from build123d import *

# Parameters (mm, degrees)
SKETCH_1_R              = 6
SKETCH_1_R_2            = 2.6
EXTRUDE_1_DEPTH         = 22
CUT_EXTRUDE_START       = -12
CUT_EXTRUDE_1_OUTLINE_R = 6
CUT_EXTRUDE_1_DEPTH     = 12
FILLET_1_R              = 5


# Read off the part's stored shape, not the designer's step: 切除-拉伸1
with BuildPart() as part:
    # 草图1 → 凸台-拉伸1 (new body)
    with BuildSketch(Plane.XY):
        with BuildLine():
            Line((24.04705584, 21.941390991), (25.62631028, -1.269568576))
            add(Edge.make_bspline(
                [(25.62631028, -1.269568576), (30.294741582, 4.490329629), (34.848985416, 10.341994574), (43.840833171, 22.214968329), (48.277316557, 28.236694952), (52.668077763, 34.291262241)],
                knots=[0.751086715, 0.751086715, 0.751086715, 0.751086715, 0.875, 0.875, 1, 1, 1, 1], degree=3))
            add(Edge.make_bspline(
                [(52.668077763, 34.291262241), (54.385569076, 36.659627804), (56.095877797, 39.033185186), (58.65356822, 42.599078019), (59.503877121, 43.78931812), (61.206685795, 46.168192958), (62.060572053, 47.355980663), (62.923151952, 48.537325445)],
                knots=[0, 0, 0, 0, 12.867122322, 12.867122322, 19.300683483, 19.300683483, 25.734244644, 25.734244644, 25.734244644, 25.734244644], degree=3))
            add(Edge.make_bspline(
                [(62.923151952, 48.537325445), (63.691030086, 49.593267388), (64.385737457, 50.528608987), (65.152866174, 51.561457391), (65.870104463, 52.500349083), (66.644032214, 53.513449395), (67.382538536, 54.446906012), (68.169071386, 55.441067159), (68.929366855, 56.362602713)],
                knots=[0, 0, 0, 0.25, 0.25, 0.5, 0.5, 0.75, 0.75, 1, 1, 1], degree=2))
            add(Edge.make_bspline(
                [(68.929366855, 56.362602713), (68.939807825, 56.376913703), (68.94904286, 56.392240586)],
                knots=[0.088106579, 0.088106579, 0.088106579, 0.143786066, 0.143786066, 0.143786066], degree=2, weights=[1, 0.999612499, 1]))
            Line((68.94904286, 56.392240586), (73.182530774, 63.58271012))
            Line((73.182530774, 63.58271012), (77.6764923, 67.17962487))
            ThreePointArc((77.6764923, 67.17962487), (78.379967095, 67.75128437), (79.091839453, 68.312452009))
            Line((79.091839453, 68.312452009), (103.36876376, 87.743421018))
            add(Edge.make_bspline(
                [(103.36876376, 87.743421018), (103.794913212, 88.083498112), (104.14591982, 88.500209303), (104.495810247, 88.915595377), (104.757584433, 89.390611784), (105.019785316, 89.866402479), (105.18387744, 90.383514181), (105.347603834, 90.89947334), (105.407790685, 91.436682712), (105.468371762, 91.977410832), (105.422168005, 92.518813243), (105.376170251, 93.057801763), (105.226513558, 93.576866403), (105.075866476, 94.099366077), (104.826403144, 94.581721125), (104.577389608, 95.06320646), (104.239613139, 95.486702432)],
                knots=[0, 0, 0, 0.125, 0.125, 0.25, 0.25, 0.375, 0.375, 0.5, 0.5, 0.625, 0.625, 0.75, 0.75, 0.875, 0.875, 1, 1, 1], degree=2))
            Line((104.239613139, 95.486702432), (102.10787197, 98.150082549))
            add(Edge.make_bspline(
                [(102.10787197, 98.150082549), (101.662660323, 98.707408746), (101.134816221, 99.186660834), (100.605787322, 99.666988651), (100.007698858, 100.056631193), (99.413800036, 100.443544268), (98.766951597, 100.73157288), (98.115443256, 101.021676452), (97.426848492, 101.204456829), (96.741213417, 101.386451586), (96.036172435, 101.457788474), (95.327397899, 101.529503128), (94.616958411, 101.487928839), (93.907956416, 101.446438671), (93.215156177, 101.29350915), (92.520746602, 101.140224382), (91.859708878, 100.879055504)],
                knots=[0, 0, 0, 0.125, 0.125, 0.25, 0.25, 0.375, 0.375, 0.5, 0.5, 0.625, 0.625, 0.75, 0.75, 0.875, 0.875, 1, 1, 1], degree=2))
            Line((91.859708878, 100.879055504), (81.022663549, 97.937140274))
            Line((81.022663549, 97.937140274), (66.880013026, 92.33227511))
            add(Edge.make_bspline(
                [(66.880013026, 92.33227511), (65.373977149, 91.735592871), (64.00578846, 90.868278931), (62.646323986, 90.006495393), (61.470305816, 88.907497765), (60.292351586, 87.806690876), (59.339427675, 86.506195587), (58.383073515, 85.201018894), (57.686838347, 83.740417625)],
                knots=[0, 0, 0, 0.25, 0.25, 0.5, 0.5, 0.75, 0.75, 1, 1, 1], degree=2))
            add(Edge.make_bspline(
                [(57.686838347, 83.740417625), (56.095548431, 80.401632953), (54.518583687, 77.162280014)],
                knots=[0, 0, 0, 1, 1, 1], degree=2))
            add(Edge.make_bspline(
                [(54.518583687, 77.162280014), (53.763269837, 75.610969128), (52.999745837, 74.063699923), (51.467519232, 70.971710828), (50.697291265, 69.427763476), (49.146563784, 66.345016376), (48.366275895, 64.806128726), (46.794629467, 61.734063391), (46.003946156, 60.200522916), (45.205011248, 58.67121375)],
                knots=[0, 0, 0, 0, 0.25, 0.25, 0.5, 0.5, 0.75, 0.75, 1, 1, 1, 1], degree=3))
            add(Edge.make_bspline(
                [(45.205011248, 58.67121375), (41.847412181, 52.245521434), (38.381271035, 45.876195204), (31.340232317, 33.621328767), (27.77883413, 27.726649653), (24.04705584, 21.941390991)],
                knots=[0, 0, 0, 0, 0.125, 0.125, 0.243696274, 0.243696274, 0.243696274, 0.243696274], degree=3))
        make_face()
        with Locations((94.625559773, 92.089088396)):
            Circle(SKETCH_1_R, mode=Mode.SUBTRACT)
        with Locations((68.602677697, 77.162280014)):
            Circle(SKETCH_1_R, mode=Mode.SUBTRACT)
        with Locations((33.14705584, 20.777472123)):
            Circle(SKETCH_1_R_2, mode=Mode.SUBTRACT)
        with Locations((57.169835175, 58.366266824)):
            Circle(SKETCH_1_R_2, mode=Mode.SUBTRACT)
    extrude(amount=EXTRUDE_1_DEPTH)

    # 切除-拉伸1 outline → 切除-拉伸1 (cut)
    with BuildSketch(Plane.XY.offset(22).offset(CUT_EXTRUDE_START)):
        with BuildLine():
            add(Edge.make_bspline(
                [(57.686838346, 83.740417623), (56.09554843, 80.401632953), (54.518583688, 77.162280014)],
                knots=[0.494428836, 0.494428836, 0.494428836, 0.494587311, 0.494587311, 0.494587311], degree=2))
            Line((54.518583688, 77.162280014), (73.182530774, 63.58271012))
            Line((73.182530774, 63.58271012), (77.6764923, 67.17962487))
            ThreePointArc((77.6764923, 67.17962487), (78.379967095, 67.75128437), (79.091839453, 68.312452009))
            Line((79.091839453, 68.312452009), (103.36876376, 87.743421018))
            add(Edge.make_bspline(
                [(103.36876376, 87.743421018), (103.794913212, 88.083498112), (104.14591982, 88.500209303), (104.495810247, 88.915595377), (104.757584433, 89.390611784), (105.019785316, 89.866402479), (105.18387744, 90.383514181), (105.347603834, 90.89947334), (105.407790685, 91.436682712), (105.468371762, 91.977410832), (105.422168005, 92.518813243), (105.376170251, 93.057801763), (105.226513558, 93.576866403), (105.075866476, 94.099366077), (104.826403144, 94.581721125), (104.577389608, 95.06320646), (104.239613139, 95.486702432)],
                knots=[0, 0, 0, 0.125, 0.125, 0.25, 0.25, 0.375, 0.375, 0.5, 0.5, 0.625, 0.625, 0.75, 0.75, 0.875, 0.875, 1, 1, 1], degree=2))
            Line((104.239613139, 95.486702432), (102.10787197, 98.150082549))
            add(Edge.make_bspline(
                [(102.10787197, 98.150082549), (101.662660323, 98.707408746), (101.134816221, 99.186660834), (100.605787322, 99.666988651), (100.007698858, 100.056631193), (99.413800036, 100.443544268), (98.766951597, 100.73157288), (98.115443256, 101.021676452), (97.426848492, 101.204456829), (96.741213417, 101.386451586), (96.036172435, 101.457788474), (95.327397899, 101.529503128), (94.616958411, 101.487928839), (93.907956416, 101.446438671), (93.215156177, 101.29350915), (92.520746602, 101.140224382), (91.859708878, 100.879055504)],
                knots=[0, 0, 0, 0.125, 0.125, 0.25, 0.25, 0.375, 0.375, 0.5, 0.5, 0.625, 0.625, 0.75, 0.75, 0.875, 0.875, 1, 1, 1], degree=2))
            Line((91.859708878, 100.879055504), (81.022663549, 97.937140274))
            Line((81.022663549, 97.937140274), (66.880013026, 92.33227511))
            add(Edge.make_bspline(
                [(66.880013026, 92.33227511), (65.373977149, 91.735592871), (64.00578846, 90.868278931), (62.646323986, 90.006495393), (61.470305816, 88.907497765), (60.292351586, 87.806690876), (59.339427675, 86.506195587), (58.383073515, 85.201018894), (57.686838346, 83.740417623)],
                knots=[0, 0, 0, 0.25, 0.25, 0.5, 0.5, 0.75, 0.75, 1, 1, 1], degree=2))
        make_face()
        with Locations((68.602677697, 77.162280014)):
            Circle(CUT_EXTRUDE_1_OUTLINE_R, mode=Mode.SUBTRACT)
        with Locations((94.625559773, 92.089088396)):
            Circle(CUT_EXTRUDE_1_OUTLINE_R, mode=Mode.SUBTRACT)
    extrude(amount=CUT_EXTRUDE_1_DEPTH, mode=Mode.SUBTRACT)

    # 圆角1
    fillet_1_edges = [part.edges().sort_by_distance(p)[0] for p in [
        (73.182530774, 63.58271012, 16),
    ]]
    fillet(fillet_1_edges, radius=FILLET_1_R)
    # the kernel refuses this fillet: 5 mm, written as the material it takes off along each edge
    with BuildSketch(Plane(origin=(54.518583687, 77.162280014, 10), x_dir=(0.8086167393984858, -0.5883357619289866, 0), z_dir=(0, 0, 1))) as fillet_1_2_piece_1:
        with BuildLine():
            CenterArc((5.939761688, -5), FILLET_1_R, 89.999999998, 99.633547548)
            Line((1.010270575, -5.836730169), (0.911680753, -5.853464772))
            ThreePointArc((0.911680753, -5.853464772), (0.412045155, -2.934442011), (-0.098457006, -0.017499087))
            Line((-0.098457006, -0.017499087), (0, 0.1))
            Line((0, 0.1), (5.939761688, 0.1))
            Line((5.939761688, 0.1), (5.939761688, 0))
        make_face()
    extrude(amount=26.849404219, mode=Mode.SUBTRACT)


solid = part.part
Geometry: final body of the model. Coordinates: model frame, mm. A direction names the side the tool comes from. Round coordinates to 2 decimals unless told otherwise and drop trailing zeros. Loops run counter-clockwise (first coordinate to the right, second up) from the corner with the lowest first, then second, coordinate; pieces in that order, holes last. Notation, with made-up numbers: M 4.5,86 L 56.5,86 A10 cw 56.5,101 Z; hole C 81.25,1 d11. An arc over 180 degrees is marked long. Put each result on its own line as item: value. Start each with the question number.
(1) Set-up query: faces 5 (the face through (64.35, 70.01, 15.92)), 6 (the face through (55.11, 56.78, 10.85)), 7 (the face through (55.248, 74.495, 15.916)). Return all of +Z, -Z, +X, -X, +Y, -Y with unobstructed straight access to the full face (end or side cutting, diameter ignored); none if empty.
(2) Draft query along X for faces 1 (the face through (100.35, 93.89, 4.93)), 2 (the face through (86.52, 99.43, 4.93)), 3 (the face through (71.477, 63.176, 16.084)), 4 (the face through (79, 84, 10)). Return one class per face: +X half, -X half, draft (parallel to the pull), parting line (faces both ways), or undercut.
(3) Section query A-A (z = 18). State how many separate pieces and enclosed holes the cut face has, then the cut area to 3 significant figures.
(4) Contact query for flat-ended pins moving along their axis: pin 1 Ø2 at (x, z) = (58.5, 17) entering from -Y; pin 2 Ø6 at (x, z) = (51, 11.5) entering from -Y; pin 3 Ø1.5 at (y, z) = (80, 6) entering from +X. Output: stop coordinate, or through.
(5) Section query B-B (x = 86). Return loops of the section in (y, z).
(6) Material intervals for line 1 along X through (y, z) = (59.5, 14.5); line 2 along Z through (x, y) = (87, 87); line 3 along X through (y, z) = (22.5, 20.75), sorted ascending. Write a range as [from, to].
Findings below:
1. face 5: +Z, +X, +Y
1. face 6: +Z, -Z
1. face 7: +Z, +Y
2. face 1: undercut
2. face 2: -X half
2. face 3: +X half
2. face 4: draft
3. separate pieces: 1
3. enclosed holes: 2
3. area: 1,280 mm2
4. pin 1: stops at y = 40.99
4. pin 2: stops at y = 27.89
4. pin 3: stops at x = 94.63
5. outline: M 73.84,0 L 99.29,0 L 99.29,10 L 73.84,10 Z
6. line 1: x = [45.64, 54.83], [59.51, 70.78]
6. line 2: z = [0, 10]
6. line 3: x = [24.41, 31.2], [35.09, 44.01]
